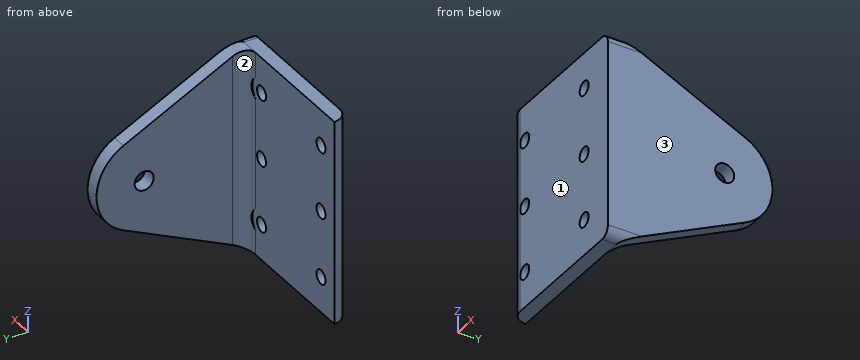
Autodesk Inventor part; units mm, degrees
ref_plane "YZ Plane" through (0, 0, 0) normal (1, 0, 0) x (0, 1, 0)
ref_plane "XZ Plane" through (0, 0, 0) normal (0, 1, 0) x (-1, 0, 0)
ref_plane "XY Plane" through (0, 0, 0) normal (0, 0, 1) x (1, 0, 0)
sketch "Szkic1" plane through (0, 0, 0) normal (0, 0, 1) x (1, 0, 0)
  line L0 (-15.1556, -3.6171) -> (-15.1556, -6.6171)
  line L1 (-15.1556, -6.6171) -> (20.8444, -6.6171)
  line L2 (20.8444, -6.6171) -> (20.8444, 40.3829)
  line L3 (20.8444, 40.3829) -> (17.8444, 40.3829)
  line L4 (17.8444, 40.3829) -> (17.8444, -3.6171)
  line L5 (17.8444, -3.6171) -> (-15.1556, -3.6171)
  point P0 (0, 0)
  dimension "d0" = 3
  dimension "d1" = 36
  dimension "d2" = 47
  dimension "d3" = 3
extrude "Wyciągnięcie proste1" add sketch "Szkic1" along normal blind 43
fillet "Zaokrąglenie1" radius 3 1 edges at (17.8444, -3.6171, 21.5)
fillet "Zaokrąglenie2" radius 3 2 edges at (-15.1556, -5.1171, 0) (-15.1556, -5.1171, 43)
sketch "Szkic3" plane through (20.8444, -6.6171, 0) normal (0, -1, 0) x (1, 0, 0)
  arc A0 (-33, 43) -> (-36, 40) centre (-33, 40) ccw
  line L0 (-36, 3) -> (-36, 40)
  arc A1 (-36, 3) -> (-33, 0) centre (-33, 3) ccw
  line L1 (-33, 0) -> (0, 0)
  line L2 (0, 0) -> (0, 43)
  line L3 (-33, 43) -> (0, 43)
  point P0 (-20.8444, 0)
  point P1 (-28, 35.5)
  point P2 (-8, 35.5)
  point P3 (-28, 7.5)
  point P4 (-8, 7.5)
  dimension "d40" = 20
  dimension "d41" = 20
  dimension "d42" = 36
  dimension "d43" = 8
  dimension "d44" = 8
  dimension "d45" = 7.5
  dimension "d46" = 7.5
  dimension "d47" = 7.5
  dimension "d48" = 7.5
hole "Otwór3" at (-7.1556, -6.6171, 35.5) at (12.8444, -6.6171, 35.5) at (-7.1556, -6.6171, 7.5) at (12.8444, -6.6171, 7.5) direction (0, 1, 0) diameter 3 end through all
sketch "Szkic4" plane through (20.8444, -6.6171, 0) normal (1, 0, 0) x (0, 0, -1)
  line L0 (0, 0) -> (0, 47)
  line L1 (0, 47) -> (-43, 47)
  line L2 (-43, 0) -> (-43, 47)
  line L3 (0, 0) -> (-43, 0)
  line L4 (0, 3) -> (-43, 3)
  circle A0 centre (-21.5, 24.5) radius 10
  line L5 (-43, 3) -> (-30.5033, 28.8521)
  line L6 (0, 3) -> (-12.4967, 28.8521)
  point P0 (0, 6.6171)
  dimension "d57" = 43
  dimension "d58" = 21.5
  dimension "d59" = 24.5
  dimension "d60" = 20
extrude "Wyciągnięcie proste4" cut sketch "Szkic4" against normal blind 10 contours L6 A0 L5 L2 L1 L0
hole "Otwór4" at (20.8444, 17.8829, 21.5) direction (-1, 0, 0) diameter 4 end through all
sketch "Szkic5" plane through (-15.1556, -3.6171, 40) normal (0, 1, 0) x (1, 0, 0)
  circle A0 centre (28, 4.5) radius 1.5
  circle A1 centre (28, 32.5) radius 1.5
  circle A2 centre (28, 4.5) radius 3.1
  circle A3 centre (28, 32.5) radius 1.5
  circle A4 centre (28, 32.5) radius 3.1
  point P0 (15.1556, 40)
  dimension "d70" = 6.2
  dimension "d71" = 6.2
extrude "Wyciągnięcie proste5" cut sketch "Szkic5" along normal blind 10
sketch "Szkic6" plane through (-15.1556, -3.6171, 40) normal (0, 1, 0) x (1, 0, 0)
  circle A0 centre (28, 4.5) radius 1.5
  circle A1 centre (28, 32.5) radius 1.5
  line L0 (30, 30.1315) -> (30, 6.8685)
  arc A2 (30, 30.1315) -> (30, 34.8685) centre (28, 32.5) ccw
  line L1 (30, 40) -> (30, 34.8685)
  line L2 (30, 40) -> (3, 40)
  arc A3 (3, 40) -> (0, 37) centre (3, 37) ccw
  line L3 (0, 37) -> (0, 0)
  arc A4 (0, 0) -> (3, -3) centre (3, 0) ccw
  line L4 (30, -3) -> (3, -3)
  line L5 (30, 2.1315) -> (30, -3)
  arc A5 (30, 2.1315) -> (30, 6.8685) centre (28, 4.5) ccw
  circle A6 centre (8, 4.5) radius 1.5
  circle A7 centre (8, 32.5) radius 1.5
  line L6 (30, 40) -> (3, 40)
  line L7 (3.5, 40) -> (3.5, -3)
  line L8 (30, -3) -> (3, -3)
  point P0 (15.1556, 40)
  dimension "d74" = 3.5
extrude "Wyciągnięcie proste6" cut sketch "Szkic6" against normal through all contours L7 L4 A4 L3 A3 L2
fillet "Zaokrąglenie3" radius 2 2 edges at (20.8444, -5.1171, 43) (20.8444, -5.1171, 0)
sketch "Szkic7" plane through (20.8444, -6.6171, 2) normal (0, -1, 0) x (1, 0, 0)
  circle A0 centre (-28, 5.5) radius 1.5
  circle A1 centre (-28, 33.5) radius 1.5
  circle A2 centre (-8, 33.5) radius 1.5
  circle A3 centre (-8, 5.5) radius 1.5
  arc A4 (-2, -2) -> (0, 0) centre (-2, 0) ccw
  line L0 (0, 0) -> (0, 39)
  arc A5 (0, 39) -> (-2, 41) centre (-2, 39) ccw
  line L1 (-32.5, 41) -> (-2, 41)
  line L2 (-32.5, 41) -> (-32.5, -2)
  line L3 (-32.5, -2) -> (-2, -2)
  point P0 (-20.8444, -2)
  point P1 (-28, 19.5)
  point P2 (-8, 19.5)
  dimension "d79" = 14
  dimension "d80" = 14
  dimension "d81" = 14
  dimension "d82" = 14
fillet "Zaokrąglenie4" radius 3 1 edges at (-11.6556, -6.6171, 21.5)
hole "Otwór5" at (-7.1556, -6.6171, 21.5) at (12.8444, -6.6171, 21.5) direction (0, 1, 0) diameter 3 end through all
properties part number "CNCM_ALU_X_Axis_Idler_Mounting_Bracket_Stiffener"
Could you check a few things on this model? Use its own coordinates, in mm. Face numbers are marked on the shaded views. Coordinates: 2 decimals unless noted, no trailing zeros. Order: outer loops, then holes, each group sorted by start corner. A loop starts at its lowest first (then second) coordinate and runs counter-clockwise, first axis right, second up.
Q1. Thinking about a two-plate mould opening in X: for the marked faces 1, 2 and 3, which applies, released by +X, released by -X, zero draft, split by the parting line, or undercut?
Q2. Please list where these lines run through material, in increasing order: L1, parallel to X at y = -5.8, z = 7.5; L2, parallel to Z at x = 12, y = -5; L3, parallel to X at y = -5.75, z = 7.5.
Q3. Will these pins go through, and if not, where does the flat tip stop? pin 1 (3 mm diameter, centred on x = 11, z = 38.5, fed in from +Y); pin 2 (1.8 mm diameter, centred on x = 12.84, z = 35.5, fed in from -Y); pin 3 (5 mm diameter, centred on y = 6.5, z = 11.5, fed in from -X); pin 4 (3.5 mm diameter, centred on x = -7.16, z = 21.5, fed in from -Y).
Q4. Suppose I cut it at B-B on x = 13.5. Please give me the cut outline in (y, z), and give its area (3 significant figures).
Q5. Suppose I cut it at A-A on z = 21.5. Give the number of separate pieces and of enclosed holes in the cut face, and give its area (3 significant figures).
Answer:
1. face 1: zero draft
1. face 2: released by -X
1. face 3: released by +X
2. L1: x = -10.71 to -8.66, -5.66 to 11.34, 14.34 to 20.84
2. L2: z = 0 to 6.26, 8.74 to 20.26, 22.74 to 34.26, 36.74 to 43
2. L3: x = -10.77 to -8.66, -5.66 to 11.34, 14.34 to 20.84
3. pin 1: stops at y = -3.62
3. pin 2: passes through
3. pin 3: stops at x = 17.84
3. pin 4: stops at y = -6.62
4. outline: (-6.62, 0) - (-3.62, 0) - (-3.62, 6.15) - (-6.62, 6.15) - close; (-6.62, 8.85) - (-3.62, 8.85) - (-3.62, 20.15) - (-6.62, 20.15) - close; (-6.62, 22.85) - (-3.62, 22.85) - (-3.62, 34.15) - (-6.62, 34.15) - close; (-6.62, 36.85) - (-3.62, 36.85) - (-3.62, 43) - (-6.62, 43) - close
4. area: 105 mm2
5. separate pieces: 4
5. enclosed holes: 0
5. area: 162 mm2
